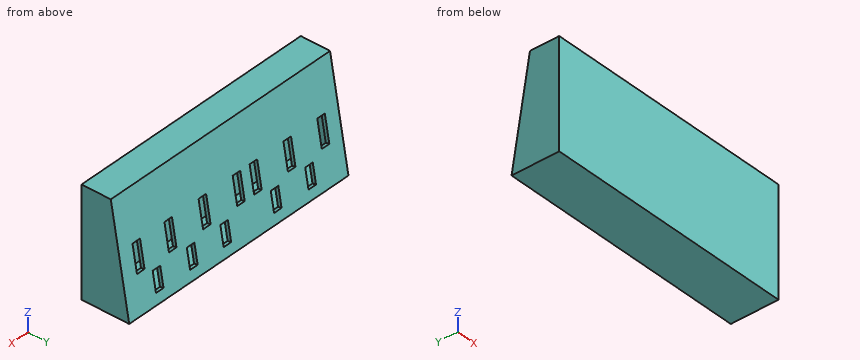
from build123d import *

# Parameters (mm, degrees)
CROQUIS1_W              = 700
CROQUIS1_H              = 298
SALIENTE_EXTRUIR1_DEPTH = 132
CORTAR_EXTRUIR1_DEPTH   = 773.158014917
CROQUIS5_W              = 24
CROQUIS5_H              = 74
CROQUIS5_H_2            = 54
CORTAR_EXTRUIR2_DEPTH   = 10
VACIADO2_START          = 10
VACIADO2_DEPTH          = 680


# Read off the part's stored shape, not the designer's step: Vaciado2
with BuildPart() as part:
    # Croquis1 → Saliente-Extruir1 (new body)
    with BuildSketch(Plane(origin=(0, 0, 0), x_dir=(1, 0, 0), z_dir=(0, 1, 0))):
        with Locations((350, 149)):
            Rectangle(CROQUIS1_W, CROQUIS1_H)
    extrude(amount=SALIENTE_EXTRUIR1_DEPTH)

    # Croquis3 → Cortar-Extruir1 (cut, through all)
    with BuildSketch(Plane.ZY):
        Polygon((0, 81), (-298, 132), (0, 132), align=None)
    extrude(amount=-CORTAR_EXTRUIR1_DEPTH, mode=Mode.SUBTRACT)

    # Croquis5 → Cortar-Extruir2 (cut)
    with BuildSketch(Plane(origin=(0, 78.695082326, 13.467950331), x_dir=(1, 0, 0), z_dir=(0, 0.9856694305119892, 0.16868839247017262))):
        with Locations((54, 180.66375979)):
            Rectangle(CROQUIS5_W, CROQUIS5_H)
        with Locations((162, 180.66375979)):
            Rectangle(CROQUIS5_W, CROQUIS5_H)
        with Locations((270, 180.66375979)):
            Rectangle(CROQUIS5_W, CROQUIS5_H)
        with Locations((324, 180.66375979)):
            Rectangle(CROQUIS5_W, CROQUIS5_H)
        with Locations((433, 180.66375979)):
            Rectangle(CROQUIS5_W, CROQUIS5_H)
        with Locations((542, 180.66375979)):
            Rectangle(CROQUIS5_W, CROQUIS5_H)
        with Locations((644, 180.66375979)):
            Rectangle(CROQUIS5_W, CROQUIS5_H)
        with Locations((110, 260.66375979)):
            Rectangle(CROQUIS5_W, CROQUIS5_H_2)
        with Locations((220, 260.66375979)):
            Rectangle(CROQUIS5_W, CROQUIS5_H_2)
        with Locations((381, 260.66375979)):
            Rectangle(CROQUIS5_W, CROQUIS5_H_2)
        with Locations((488, 260.66375979)):
            Rectangle(CROQUIS5_W, CROQUIS5_H_2)
        with Locations((597, 260.66375979)):
            Rectangle(CROQUIS5_W, CROQUIS5_H_2)
    extrude(amount=-CORTAR_EXTRUIR2_DEPTH, mode=Mode.SUBTRACT)

    # Vaciado2 outline → Vaciado2 (cut)
    with BuildSketch(Plane.YZ.offset(VACIADO2_START)):
        Polygon((93.072796716, -129.823909891), (72.566020191, -10), (10, -10), (10, -288), (120.143201399, -288), (117.363925232, -271.760307885), (108.254752038, -218.534158637), (105.555737759, -202.763447749), align=None)
    extrude(amount=VACIADO2_DEPTH, mode=Mode.SUBTRACT)


solid = part.part
Model file for the job. Use its own axes, mm. Give positions to 0.01 mm unless a question says otherwise; leave off trailing zeros. Write each loop counter-clockwise with the first axis right and the second up, starting at its lowest first coordinate (ties: lowest second). Pieces come first, ordered by that corner, then holes. Notation, with made-up numbers: (43.25, -24) -> (58.25, -24) arc R9 ccw to (58.25, -20) -> close; hole circle Ø3 at (82.5, 39.5). An arc over 180 degrees is marked (long way). Write item = value, one per line.
(1) Slice it at A-A, the plane y = 24.5. Give the cut face in (x, z).
Determined:
outline = (0, -298) -> (700, -298) -> (700, 0) -> (0, 0) -> close; hole (10, -288) -> (690, -288) -> (690, -10) -> (10, -10) -> close
(2) Probe line 1 along X through (y, z) = (21, -32.5); line 2 along X through (y, z) = (118.5, -267); line 3 along Z through (x, y) = (246.5, 19). List the from-to ranges inside material, lowest first.
Determined:
line_1 = 0 to 10, 690 to 700
line_2 = 0 to 98, 122 to 208, 232 to 369, 393 to 476, 500 to 585, 609 to 700
line_3 = -298 to -288, -10 to 0
(3) Slice it at C-C, the plane z = -114. Give the cut face in (x, y), then the cut area to 3 significant figures.
Determined:
outline = (0, 0) -> (700, 0) -> (700, 100.51) -> (0, 100.51) -> close; hole (10, 10) -> (690, 10) -> (690, 90.36) -> (10, 90.36) -> close
area = 15,700 mm2
(4) Flat gauge pin, fed straight in: P1, Ø1, axis at x = 435.5, z = -144, coming from the +Y side. Where does the tip first touch, or does it go through?
Determined:
P1 = 10
(5) Slice it at D-D, the plane z = -243. Give the cut face in (x, y), then the cut area to 3 significant figures.
Determined:
outline = (0, 0) -> (700, 0) -> (700, 122.59) -> (609, 122.59) -> (609, 112.44) -> (690, 112.44) -> (690, 10) -> (10, 10) -> (10, 112.44) -> (98, 112.44) -> (98, 122.59) -> (0, 122.59) -> close; (122, 112.44) -> (208, 112.44) -> (208, 122.59) -> (122, 122.59) -> close; (232, 112.44) -> (369, 112.44) -> (369, 122.59) -> (232, 122.59) -> close; (393, 112.44) -> (476, 112.44) -> (476, 122.59) -> (393, 122.59) -> close; (500, 112.44) -> (585, 112.44) -> (585, 122.59) -> (500, 122.59) -> close
area = 14,900 mm2
(6) Slice it at B-B, the plane x = 133. Give the cut face in (y, z).
Determined:
outline = (0, -298) -> (132, -298) -> (81, 0) -> (0, 0) -> close; hole (10, -288) -> (120.14, -288) -> (72.57, -10) -> (10, -10) -> close
